from build123d import *

# Parameters (mm, degrees)
EXTRUDE_1_DEPTH          = 10
CUT_EXTRUDE_1_DEPTH      = 38.416573868
CUT_EXTRUDE_1_DEPTH_BACK = 38.416573868
SKETCH_3_W               = 15.208425039
SKETCH_3_H               = 10


with BuildPart() as part:
    # 草图2 → 凸台-拉伸1 (new, symmetric)
    with BuildSketch(Plane(origin=(0, 0, 0), x_dir=(1, 0, 0), z_dir=(0, 1, 0))):
        with BuildLine():
            Line((11.180339887, 10), (30, 10))
            Line((30, 10), (30, -10))
            Line((30, -10), (11.180339887, -10))
            ThreePointArc((11.180339887, -10), (15, 0), (11.180339887, 10))
        make_face()
    extrude(amount=EXTRUDE_1_DEPTH, both=True)

    # 草图3 → 切除-拉伸1 (cut, two sides: drawn at the far end of the back side and taken through both)
    with BuildSketch(Plane.XY.offset(10).offset(-CUT_EXTRUDE_1_DEPTH_BACK)):
        with Locations((27.60421252, 0)):
            Rectangle(SKETCH_3_W, SKETCH_3_H)
    extrude(amount=CUT_EXTRUDE_1_DEPTH + CUT_EXTRUDE_1_DEPTH_BACK, mode=Mode.SUBTRACT)


solid = part.part
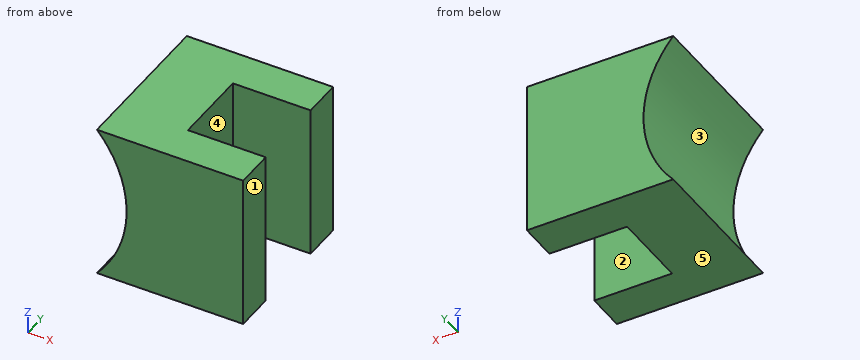
The model under review builds one solid part; all positions refer to its coordinate system, in mm. Face numbers are marked on the shaded views. A direction names the side the tool comes from. Round coordinates to 2 decimals unless told otherwise and drop trailing zeros. Loops run counter-clockwise (first coordinate to the right, second up) from the corner with the lowest first, then second, coordinate; pieces in that order, holes last. Notation, with made-up numbers: M 67,48 L 98,48 A20 ccw 98,78 Z; hole C 36.25,33.5 d8. An arc over 180 degrees is marked long. Answer as CSV lines item,"result". Start each with the question number.
Item 1: For the marked faces 1 and 2, list the 3-axis set-ups (+Z, -Z, +X, -X, +Y, -Y) from which the entire face can be reached by the end or side of a thin tool; tool diameter is ignored.
Item 2: Consider section C-C (y = -7.75). Write out the cut boundary in (x, z), then the cut area to 3 significant figures.
Item 3: Consider section D-D (x = 26.75). Write out the cut boundary in (y, z), then the cut area to 3 significant figures.
Item 4: Mouldability with a two-part tool opening along Z and no side actions: class the marked faces 3, 4 and 5 as released by +Z, released by -Z, zero draft, split by the parting line, or undercut.
Item 5: Wall thickness on line 1 (Y direction, x = 28.5, z = 7); line 2 (Z direction, x = 12.5, y = -6.75); line 3 (Z direction, x = 13.25, y = 8.75): over which ranges is each line inside the solid? List them lowest first. Write a range as [from, to].
Item 6: Insertion check: P1, Ø10, axis at y = -4.5, z = 2.5, coming from the -X side; P2, Ø1.5, axis at y = -5, z = -0.5, coming from the -X side; P3, Ø3, axis at y = 7.5, z = 8, coming from the -X side. Each pin has a flat end and moves straight along its axis. Give the tip position at first contact, or say it passes through.
Item 7: Consider section B-B (z = 2). Write out the cut boundary in (x, y).
Item 8: Consider section A-A (x = 14.5). Write out the cut boundary in (y, z), then the cut area to 3 significant figures.
Answer:
1,face 1,"+Z, -Z, +X, +Y, -Y"
1,face 2,"+Z, -Z, +X"
2,outline,"M 11.18,-10 L 30,-10 L 30,10 L 11.18,10 A15 cw Z"
2,area,"324 mm^2"
3,outline,"M -10,-10 L -5,-10 L -5,10 L -10,10 Z; M 5,-10 L 10,-10 L 10,10 L 5,10 Z"
3,area,"200 mm^2"
4,face 3,"undercut"
4,face 4,"zero draft"
4,face 5,"released by -Z"
5,line 1,"y = [-10, -5], [5, 10]"
5,line 2,"z = [-10, -8.29], [8.29, 10]"
5,line 3,"z = [-10, -7.03], [7.03, 10]"
6,P1,"stops at x = 12.99"
6,P2,"stops at x = 14.95"
6,P3,"stops at x = 11.61"
7,outline,"M 14.87,-10 L 30,-10 L 30,-5 L 20,-5 L 20,5 L 30,5 L 30,10 L 14.87,10 Z"
8,outline,"M -10,-10 L 10,-10 L 10,-3.84 L -10,-3.84 Z; M -10,3.84 L 10,3.84 L 10,10 L -10,10 Z"
8,area,"246 mm^2"
